```python
from build123d import *

# Parameters (mm, degrees)
CYLINDER053_R      = 2.5
CYLINDER053_DEPTH  = 50
CYLINDER052_R      = 4.8
CYLINDER052_DEPTH  = 28
CHAMFER006009_SIZE = 1
CHAMFER006010_SIZE = 0.6


with BuildPart() as cylinder063:
    # Cylinder053 → Cylinder053 (new body)
    with BuildSketch(Plane.XY.offset(-4)):
        Circle(CYLINDER053_R)
    extrude(amount=CYLINDER053_DEPTH)


with BuildPart() as locating_cylinder:
    # Cylinder052 → Cylinder052 (new body)
    with BuildSketch(Plane.XY):
        Circle(CYLINDER052_R)
    extrude(amount=CYLINDER052_DEPTH)

    # Cut144: cut Cylinder063
    add(cylinder063.part, mode=Mode.SUBTRACT)


with BuildPart() as locating_cylinder_1:
    # Cut144 placement: moved
    add(locating_cylinder.part.moved(Location((-6, 33, 0))))

    # Chamfer006009
    chamfer006009_edges = [locating_cylinder_1.edges().sort_by_distance(p)[0] for p in [
        (-10.8, 33, 28),
    ]]
    chamfer(chamfer006009_edges, length=CHAMFER006009_SIZE)

    # Chamfer006010
    chamfer006010_edges = [locating_cylinder_1.edges().sort_by_distance(p)[0] for p in [
        (-10.8, 33, 0),
    ]]
    chamfer(chamfer006010_edges, length=CHAMFER006010_SIZE)


solid = locating_cylinder_1.part
```
Could you check a few things on this model? Use its own coordinates, in mm. Round coordinates to 2 decimals unless told otherwise and drop trailing zeros. Loops run counter-clockwise (first coordinate to the right, second up) from the corner with the lowest first, then second, coordinate; pieces in that order, holes last. Notation, with made-up numbers: (-4.75, -20.75) - (49.25, -20.75) arc R21 ccw to (49.25, -13.75) - close; hole circle Ø4 at (35, -34). An arc over 180 degrees is marked (long way). Answer as CSV lines item,"result".
1. I want a section at A-A on y = 33. List the corners of the cut face in (x, z) for me, then the cut area to 3 significant figures.
Filled in:
outline,"(-10.8, 0.6) - (-10.2, 0) - (-8.5, 0) - (-8.5, 28) - (-9.8, 28) - (-10.8, 27) - close; (-3.5, 0) - (-1.8, 0) - (-1.2, 0.6) - (-1.2, 27) - (-2.2, 28) - (-3.5, 28) - close"
area,"127 mm^2"
2. For pin 1 Ø4 at (x, y) = (-6, 33) entering from -Z; pin 2 Ø4 at (y, z) = (35.5, 5.5) entering from +X; pin 3 Ø2 at (x, z) = (-9.5, 7.5) entering from -Y; pin 4 Ø5 at (x, z) = (-9.5, 21.5) entering from +Y, each with a flat end and sliding along its axis, tell me the tip position at first contact or that it passes through.
Filled in:
pin 1,"passes through"
pin 2,"stops at x = -1.23"
pin 3,"stops at y = 28.9"
pin 4,"stops at y = 37.69"
3. We'd pull the mould along X, two halves only. Please class faces 1 (the face through (-4, 31, 0)), 2 (the face through (-4.66, 35.11, 13.8)), 3 (the face through (-9.81, 30.08, 13.62)): +X half, -X half, draft (parallel to the pull), parting line (faces both ways), or undercut.
Filled in:
face 1,"draft"
face 2,"undercut"
face 3,"parting line"
4. I want a section at B-B on x = -6. List the corners of the cut face in (y, z) for me.
Filled in:
outline,"(28.2, 0.6) - (28.8, 0) - (30.5, 0) - (30.5, 28) - (29.2, 28) - (28.2, 27) - close; (35.5, 0) - (37.2, 0) - (37.8, 0.6) - (37.8, 27) - (36.8, 28) - (35.5, 28) - close"
5. Please list where these lines run through material, in increasing order: line 1 along Y through (x, z) = (-6, 13.5); line 2 along X through (y, z) = (32, 3.5); line 3 along Y through (x, z) = (-8, 7.75). Write a range as [from, to].
Filled in:
line 1,"y = [28.2, 30.5], [35.5, 37.8]"
line 2,"x = [-10.69, -8.29], [-3.71, -1.31]"
line 3,"y = [28.64, 31.5], [34.5, 37.36]"
6. I want a section at C-C on z = 15.25. List the corners of the cut face in (x, y) for me, then the cut area to 3 significant figures.
Filled in:
outline,"circle Ø9.6 at (-6, 33); hole circle Ø5 at (-6, 33)"
area,"52.7 mm^2"
